Read the model definition and answer for the solid it produces. Units are mm, in the model's axes. A direction names the side the tool comes from. Round coordinates to 2 decimals unless told otherwise and drop trailing zeros. Order: outer loops, then holes, each group sorted by start corner. A loop starts at its lowest first (then second) coordinate and runs counter-clockwise, first axis right, second up. Notation, with made-up numbers: (67.5, -36) -> (113.5, -36) arc R27 cw to (113.5, 0) -> close; hole circle Ø10 at (88.25, 20.25). An arc over 180 degrees is marked (long way). Answer as a JSON object with one key per item and string values. Group by question number.
Item 1: Consider probe 1 along Y at (x, z) = (6, -27.5); probe 2 along Y at (x, z) = (17, -33.5); probe 3 along Z at (x, y) = (-10.5, 3.5). Determine where each line is inside the solid, lowest interval first. Write a range as from..to.
Item 2: For faces 1 (the cylindrical face through (-0.46, 13.45, -47.22)), 2 (the flat face through (30, 20, -10)), 3 (the flat face through (31, 17, 31)), 4 (the flat face through (0, 17, -44)), determine the directions among +Z, -Z, +X, -X, +Y, -Y from which every point of the face is accessible in a straight line to the end or side of a thin tool.
Item 3: Section C-C, the plane y = 3.5 is taken. Write down the section's boundary in (x, z).
Item 4: Section D-D, the plane y = -13 is taken. Write down the section's boundary in (x, z), plus the area to 3 significant figures.
Item 5: Given P1, Ø5.5, axis at x = -31, z = -31.5, coming from the +Y side; P2, Ø1.5, axis at x = -10, z = 14.5, coming from the -Y side; P3, Ø1, axis at x = -2.5, y = -15.5, coming from the -Z side; P4, Ø21.5, axis at x = 0.5, z = 9, coming from the +Y side, each flat-ended and moving along its own axis, determine where each tip first touches the part or whether it passes through.
Item 6: Section B-B, the plane z = 0 is taken. Write down the section's boundary in (x, y).
Item 7: Section A-A, the plane x = 0 is taken. Write down the section's boundary in (y, z).
Item 8: The mould has two halves that part along Z. Classify faces 5 (the flat face through (0, 17, 44)), 6 (the cylindrical face through (-14.57, 18.48, 30.62)), 7 (the cylindrical face through (-22.818, 12.465, -29.759)): pulls with the +Z half, pulls with the -Z half, needs draft (parallel to the pull), parting line crosses it, or undercut.
from build123d import *

# Parameters (mm, degrees)
SKETCH2_R                = 50
BOSS_EXTRUDE1_DEPTH      = 10
SKETCH4_R                = 37.5
BOSS_EXTRUDE3_DEPTH      = 7
SKETCH5_R                = 3.5
BOSS_EXTRUDE4_DEPTH      = 7
CIRPATTERN1_COUNT        = 8
SKETCH6_R                = 2
BOSS_EXTRUDE5_DEPTH      = 3
CIRPATTERN2_COUNT        = 8
CHAMFER1_SIZE            = 2
FILLET1_R                = 2
BOSS_EXTRUDE6_DEPTH      = 20
BOSS_EXTRUDE6_DEPTH_BACK = 20
SKETCH7_R                = 7.5


with BuildPart() as part:
    # Sketch2 → Boss-Extrude1 (new body)
    with BuildSketch(Plane(origin=(0, 0, 0), x_dir=(1, 0, 0), z_dir=(0, 1, 0))):
        with Locations(Location((0, 0, 0), (0, 0, 270))):
            Circle(SKETCH2_R)
    extrude(amount=BOSS_EXTRUDE1_DEPTH)

    # Sketch4 → Boss-Extrude3 (add)
    with BuildSketch(Plane(origin=(0, 10, 0), x_dir=(1, 0, 0), z_dir=(0, 1, 0))):
        with Locations(Location((0, 0, 0), (0, 0, 270))):
            Circle(SKETCH4_R)
    extrude(amount=BOSS_EXTRUDE3_DEPTH)

    # Sketch5 → Boss-Extrude4 (add)
    with BuildSketch(Plane(origin=(0, 10, 0), x_dir=(1, 0, 0), z_dir=(0, 1, 0))):
        with Locations(Location((43.75, 0, 0), (0, 0, 270))):
            Circle(SKETCH5_R)
    boss_extrude4 = extrude(amount=BOSS_EXTRUDE4_DEPTH)

    # CirPattern1: Boss-Extrude4 ×8 about axis
    cirpattern1_axis = Axis((0, 0, 0), (0, 1, 0))
    for i in range(1, CIRPATTERN1_COUNT):
        add(boss_extrude4.rotate(cirpattern1_axis, i * 360 / CIRPATTERN1_COUNT))

    # Sketch6 → Boss-Extrude5 (add)
    with BuildSketch(Plane(origin=(0, 17, 0), x_dir=(1, 0, 0), z_dir=(0, 1, 0))):
        with Locations(Location((30.433808521, 9.88854382, 0), (0, 0, 270))):
            Circle(SKETCH6_R)
    boss_extrude5 = extrude(amount=BOSS_EXTRUDE5_DEPTH)

    # CirPattern2: Boss-Extrude5 ×8 about axis
    cirpattern2_axis = Axis((-0.086814216, 0, 0.028207649), (0, 1, 0))
    for i in range(1, CIRPATTERN2_COUNT):
        add(boss_extrude5.rotate(cirpattern2_axis, i * 360 / CIRPATTERN2_COUNT))

    # Chamfer1
    chamfer1_edges = [part.edges().sort_by_distance(p)[0] for p in [
        (0, 17, -37.5),
    ]]
    chamfer(chamfer1_edges, length=CHAMFER1_SIZE)

    # Fillet1
    fillet1_edges = [part.edges().sort_by_distance(p)[0] for p in [
        (0, 10, -50),
    ]]
    fillet(fillet1_edges, radius=FILLET1_R)

    # Sketch7 → Boss-Extrude6 (add, two sides: drawn at the far end of the back side and taken through both)
    with BuildSketch(Plane.XZ.offset(-BOSS_EXTRUDE6_DEPTH_BACK)):
        with Locations(Location((0, 0, 0), (0, 0, 270))):
            Circle(SKETCH7_R)
    extrude(amount=BOSS_EXTRUDE6_DEPTH + BOSS_EXTRUDE6_DEPTH_BACK)


solid = part.part
Values found:
{
 "1": {"probe 1": "0..17", "probe 2": "0..10", "probe 3": "-48.89..48.89"},
 "2": {"face 1": "+Y", "face 2": "+Z, -Z, +X, -X, +Y", "face 3": "+Z, +X, +Y", "face 4": "-Z, +X, -X, +Y"},
 "3": {"outline": "circle Ø100 at (0, 0)"},
 "4": {"outline": "circle Ø15 at (0, 0)", "area": "177 mm2"},
 "5": {"P1": "y = 17", "P2": "y = 0", "P3": "z = -7.23", "P4": "y = 20"},
 "6": {"outline": "(-50, 0) -> (-7.5, 0) -> (-7.5, -20) -> (7.5, -20) -> (7.5, 0) -> (50, 0) -> (50, 8) arc R2 ccw to (48, 10) -> (47.25, 10) -> (47.25, 17) -> (40.25, 17) -> (40.25, 10) -> (37.5, 10) -> (37.5, 15) -> (35.5, 17) -> (7.5, 17) -> (7.5, 20) -> (-7.5, 20) -> (-7.5, 17) -> (-35.5, 17) -> (-37.5, 15) -> (-37.5, 10) -> (-40.25, 10) -> (-40.25, 17) -> (-47.25, 17) -> (-47.25, 10) -> (-48, 10) arc R2 ccw to (-50, 8) -> close"},
 "7": {"outline": "(-20, -7.5) -> (0, -7.5) -> (0, -50) -> (8, -50) arc R2 ccw to (10, -48) -> (10, -47.25) -> (17, -47.25) -> (17, -40.25) -> (10, -40.25) -> (10, -37.5) -> (15, -37.5) -> (17, -35.5) -> (17, -7.5) -> (20, -7.5) -> (20, 7.5) -> (17, 7.5) -> (17, 35.5) -> (15, 37.5) -> (10, 37.5) -> (10, 40.25) -> (17, 40.25) -> (17, 47.25) -> (10, 47.25) -> (10, 48) arc R2 ccw to (8, 50) -> (0, 50) -> (0, 7.5) -> (-20, 7.5) -> close"},
 "8": {"face 5": "needs draft", "face 6": "parting line crosses it", "face 7": "undercut"}
}
